Print and shaded views of the part. All mm, measured from the part's lowest x, y and z. A direction names the side the tool comes from. Round coordinates to 2 decimals unless told otherwise and drop trailing zeros. Write each loop counter-clockwise with the first axis right and the second up, starting at its lowest first coordinate (ties: lowest second). Pieces come first, ordered by that corner, then holes. Notation, with made-up numbers: M 65.25,-32.5 L 75.25,-32.5 A14 cw 75.25,-5.5 Z; hole C 16.25,-33 d10. An arc over 180 degrees is marked long. Write item = value, one per line.
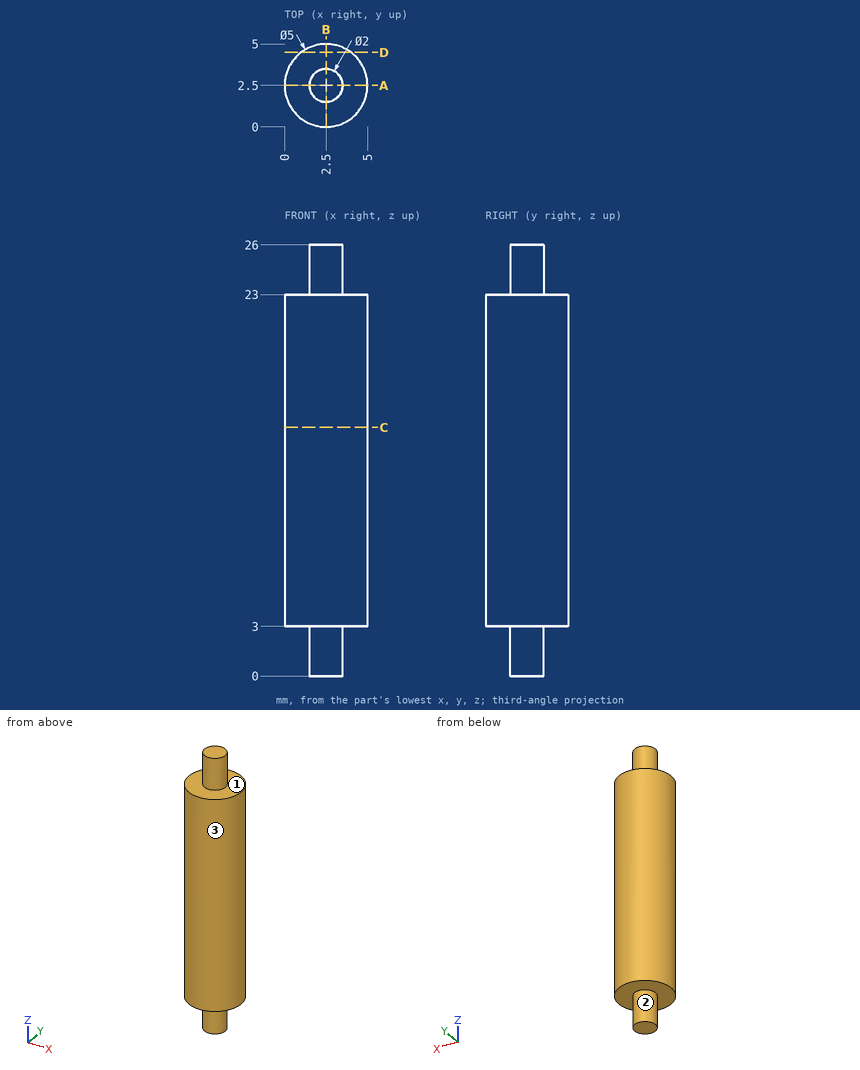
1. Band-saw the part on C-C (z = 15). List the corners of the cut face in (x, y).
Responses:
outline = C 2.5,2.5 d5
2. Tool access for the marked faces 1, 2 and 3: list every direction of +Z, -Z, +X, -X, +Y, -Y with a clear straight run to the whole face (end or side of a thin tool).
Responses:
face_1 = +Z
face_2 = -Z
face_3 = +Z, -Z
3. Probe probe 1 along Z at (x, y) = (3.3, 4.3); probe 2 along Y at (x, z) = (2.4, 3.5); probe 3 along X at (y, z) = (1.1, 16.75). List the from-to ranges inside material, lowest first.
Responses:
probe_1 = 3 to 23
probe_2 = 0 to 5
probe_3 = 0.43 to 4.57
4. Flat gauge pins, fed straight in: pin 1 (1 mm diameter, centred on y = 1.5, z = 10.5, fed in from +X); pin 2 (1 mm diameter, centred on x = 3.5, y = 1, fed in from -Z). Where does each tip first touch, or does it go through?
Responses:
pin_1 = 4.95
pin_2 = 3
5. Band-saw the part on A-A (y = 2.5). List the corners of the cut face in (x, z).
Responses:
outline = M 0,3 L 1.5,3 L 1.5,0 L 3.5,0 L 3.5,3 L 5,3 L 5,23 L 3.5,23 L 3.5,26 L 1.5,26 L 1.5,23 L 0,23 Z
6. Band-saw the part on D-D (y = 4.5). List the corners of the cut face in (x, z), plus the area to 3 significant figures.
Responses:
outline = M 1,3 L 4,3 L 4,23 L 1,23 Z
area = 60.0 mm²
